from build123d import *

# Parameters (mm, degrees)
BOSS_EXTRUDE1_DEPTH                            = 27.5
CBORE_FOR_M3_SBHCS1_D                          = 3.4
CBORE_FOR_M3_SBHCS1_DEPTH                      = 14.9999954
CBORE_FOR_M3_SBHCS1_CBORE_D                    = 6.7
CBORE_FOR_M3_SBHCS1_CBORE_DEPTH                = 1.65
CBORE_FOR_M3_SBHCS1_TIP                        = 1.021463052
SKETCH4_W                                      = 41.25
SKETCH4_H                                      = 7.273611758
BOSS_EXTRUDE2_DEPTH                            = 4.5
CSK_FOR_M5_FLAT_HEAD_MACHINE_SCREW1_AT_2_COUNT = 2
CSK_FOR_M5_FLAT_HEAD_MACHINE_SCREW1_AT_2_PITCH = 32
CSK_FOR_M5_FLAT_HEAD_MACHINE_SCREW1_AT_3_COUNT = 2
CSK_FOR_M5_FLAT_HEAD_MACHINE_SCREW1_AT_3_PITCH = 43.863424399
CSK_FOR_M5_FLAT_HEAD_MACHINE_SCREW1_AT_4_COUNT = 2
CSK_FOR_M5_FLAT_HEAD_MACHINE_SCREW1_AT_4_PITCH = 30
CUT_EXTRUDE1_REACH                             = 136.892
CUT_EXTRUDE1_END_RADIUS                        = 57.15
SKETCH13_R                                     = 5.2
CHAMFER1_START                                 = -27.5
CHAMFER1_DEPTH                                 = 55
CHAMFER1_START_2                               = -3.038209282
CHAMFER1_2_OUTLINE_R                           = 3.35
CHAMFER1_2_DEPTH                               = 1.570474688
CHAMFER2_SIZE                                  = 1


with BuildPart() as part:
    # Sketch1 → Boss-Extrude1 (new, symmetric)
    with BuildSketch(Plane(origin=(0, 0, 0), x_dir=(1, 0, 0), z_dir=(0, 1, 0))):
        with BuildLine():
            Line((-25.625, 54.611949242), (-25.625, 69.598611758))
            Line((-25.625, 69.598611758), (-20.625, 69.598611758))
            Line((-20.625, 69.598611758), (-20.625, 62.325))
            Line((-20.625, 62.325), (20.625, 62.325))
            Line((20.625, 62.325), (20.625, 69.598611758))
            Line((20.625, 69.598611758), (25.625, 69.598611758))
            Line((25.625, 69.598611758), (28.64505971, 67.064480768))
            Line((28.64505971, 67.064480768), (21.893060118, 59.017760997))
            Line((21.893060118, 59.017760997), (25.723282334, 55.803822949))
            Line((25.723282334, 55.803822949), (32.475281926, 63.85054272))
            Line((32.475281926, 63.85054272), (36.305504142, 60.636604672))
            Line((36.305504142, 60.636604672), (29.553504549, 52.5898849))
            Line((29.553504549, 52.5898849), (31.287947409, 47.824542307))
            ThreePointArc((31.287947409, 47.824542307), (-32.73018113, -46.849308887), (34.142039673, 45.830597061))
            Line((34.142039673, 45.830597061), (32.272757303, 50.966408163))
            Line((32.272757303, 50.966408163), (38.7006334, 58.626852595))
            Line((38.7006334, 58.626852595), (42.530855615, 55.412914546))
            Line((42.530855615, 55.412914546), (36.399549462, 48.10590841))
            ThreePointArc((36.399549462, 48.10590841), (-6.293240092, -59.995839474), (-25.625, 54.611949242))
        make_face()
    extrude(amount=BOSS_EXTRUDE1_DEPTH, both=True)

    # CBORE for M3 SBHCS1
    with Locations(Plane(origin=(-2.327403337, 0, -1.952923282), x_dir=(0.6427876096865344, 0, -0.7660444431189822), z_dir=(0.7660444431189822, 0, 0.6427876096865344))):
        with Locations((65.056031142, 20), (65.056031142, 0), (65.056031142, -20)):
            CounterBoreHole(CBORE_FOR_M3_SBHCS1_D / 2, CBORE_FOR_M3_SBHCS1_CBORE_D / 2, CBORE_FOR_M3_SBHCS1_CBORE_DEPTH, depth=CBORE_FOR_M3_SBHCS1_DEPTH)
            with Locations((0, 0, -(CBORE_FOR_M3_SBHCS1_DEPTH + CBORE_FOR_M3_SBHCS1_TIP / 2))):  # 118° drill point
                Cone(0, CBORE_FOR_M3_SBHCS1_D / 2, CBORE_FOR_M3_SBHCS1_TIP, mode=Mode.SUBTRACT)

    # Sketch4 → Boss-Extrude2 (add)
    with BuildSketch(Plane.XZ.offset(-27.5)):
        with Locations((0, -65.961805879)):
            Rectangle(SKETCH4_W, SKETCH4_H)
    extrude(amount=BOSS_EXTRUDE2_DEPTH)

    # Sketch12 → CSK for M5 Flat Head Machine Screw1 (revolve, cut)
    with BuildSketch(Plane(origin=(-16, 15, -57.15), x_dir=(0, -1, 0), z_dir=(1, 0, 0))):
        Polygon((0, 0), (0, 12.448611758), (2.75, 12.448611758), (2.75, 2.45), (5.2, 0), align=None)
    csk_for_m5_flat_head_machine_screw1 = revolve(axis=Axis((-16, 15, -50.8), (0, 0, -1)), mode=Mode.SUBTRACT)

    # CSK for M5 Flat Head Machine Screw1 at 2: CSK for M5 Flat Head Machine Screw1 ×2
    with Locations(*[(i * CSK_FOR_M5_FLAT_HEAD_MACHINE_SCREW1_AT_2_PITCH, 0, 0) for i in range(1, CSK_FOR_M5_FLAT_HEAD_MACHINE_SCREW1_AT_2_COUNT)]):
        add(csk_for_m5_flat_head_machine_screw1, mode=Mode.SUBTRACT)

    # CSK for M5 Flat Head Machine Screw1 at 3: CSK for M5 Flat Head Machine Screw1 ×2
    with Locations(*[Vector(0.7295372041400852, -0.6839411288813297, 0) * (i * CSK_FOR_M5_FLAT_HEAD_MACHINE_SCREW1_AT_3_PITCH) for i in range(1, CSK_FOR_M5_FLAT_HEAD_MACHINE_SCREW1_AT_3_COUNT)]):
        add(csk_for_m5_flat_head_machine_screw1, mode=Mode.SUBTRACT)

    # CSK for M5 Flat Head Machine Screw1 at 4: CSK for M5 Flat Head Machine Screw1 ×2
    with Locations(*[(0, -i * CSK_FOR_M5_FLAT_HEAD_MACHINE_SCREW1_AT_4_PITCH, 0) for i in range(1, CSK_FOR_M5_FLAT_HEAD_MACHINE_SCREW1_AT_4_COUNT)]):
        add(csk_for_m5_flat_head_machine_screw1, mode=Mode.SUBTRACT)

    # Cut-Extrude1: up to this cylinder (the profile starts outside it)
    cut_extrude1_end = Plane(origin=(0, 0, 0), z_dir=(0, -1, 0)) * Cylinder(CUT_EXTRUDE1_END_RADIUS, 419.084, mode=Mode.PRIVATE)
    # Sketch13 → Cut-Extrude1 (cut, up to the surface)
    with BuildSketch(Plane.XY.offset(-57.15), mode=Mode.PRIVATE) as cut_extrude1_sk1:
        with Locations(Location((-16, -15, 0), (0, 0, 180))):
            Circle(SKETCH13_R)
    cut_extrude1_tool1 = extrude(cut_extrude1_sk1.sketch, amount=CUT_EXTRUDE1_REACH, mode=Mode.PRIVATE) - cut_extrude1_end
    add(cut_extrude1_tool1.solids().sort_by_distance((-16, -15, -57.15))[0], mode=Mode.SUBTRACT)
    # Sketch13 → Cut-Extrude1 (cut, up to the surface)
    with BuildSketch(Plane.XY.offset(-57.15), mode=Mode.PRIVATE) as cut_extrude1_sk2:
        with Locations(Location((16, -15, 0), (0, 0, 180))):
            Circle(SKETCH13_R)
    cut_extrude1_tool2 = extrude(cut_extrude1_sk2.sketch, amount=CUT_EXTRUDE1_REACH, mode=Mode.PRIVATE) - cut_extrude1_end
    add(cut_extrude1_tool2.solids().sort_by_distance((16, -15, -57.15))[0], mode=Mode.SUBTRACT)
    # Sketch13 → Cut-Extrude1 (cut, up to the surface)
    with BuildSketch(Plane.XY.offset(-57.15), mode=Mode.PRIVATE) as cut_extrude1_sk3:
        with Locations(Location((16, 15, 0), (0, 0, 180))):
            Circle(SKETCH13_R)
    cut_extrude1_tool3 = extrude(cut_extrude1_sk3.sketch, amount=CUT_EXTRUDE1_REACH, mode=Mode.PRIVATE) - cut_extrude1_end
    add(cut_extrude1_tool3.solids().sort_by_distance((16, 15, -57.15))[0], mode=Mode.SUBTRACT)
    # Sketch13 → Cut-Extrude1 (cut, up to the surface)
    with BuildSketch(Plane.XY.offset(-57.15), mode=Mode.PRIVATE) as cut_extrude1_sk4:
        with Locations(Location((-16, 15, 0), (0, 0, 180))):
            Circle(SKETCH13_R)
    cut_extrude1_tool4 = extrude(cut_extrude1_sk4.sketch, amount=CUT_EXTRUDE1_REACH, mode=Mode.PRIVATE) - cut_extrude1_end
    add(cut_extrude1_tool4.solids().sort_by_distance((-16, 15, -57.15))[0], mode=Mode.SUBTRACT)

    # Chamfer1: read off the stored shape, not the designer's step
    # Chamfer1 outline → Chamfer1 (add)
    with BuildSketch(Plane(origin=(0, 0, 0), x_dir=(1, 0, 0), z_dir=(0, 1, 0)).offset(CHAMFER1_START)):
        with BuildLine():
            ThreePointArc((36.399549462, 48.10590841), (37.595386052, 47.177246344), (38.767539596, 46.218865181))
            Line((38.767539596, 46.218865181), (38.293658487, 50.363219646))
            Line((38.293658487, 50.363219646), (36.399549462, 48.10590841))
        make_face()
        with BuildLine():
            Line((-25.625, 57.786949242), (-32.752511971, 50.659437271))
            ThreePointArc((-32.752511971, 50.659437271), (-29.255581753, 52.756199269), (-25.625, 54.611949242))
            Line((-25.625, 54.611949242), (-25.625, 57.786949242))
        make_face()
    extrude(amount=CHAMFER1_DEPTH)

    # Chamfer1 2 outline → Chamfer1 2 (cut)
    with BuildSketch(Plane(origin=(0, 0, 0), x_dir=(0.642787609686534, 0, -0.7660444431189825), z_dir=(0.7660444431189823, 0, 0.6427876096865344)).offset(CHAMFER1_START_2)):
        with Locations((65.056031142, -20)):
            Circle(CHAMFER1_2_OUTLINE_R)
        with Locations((65.056031142, 0)):
            Circle(CHAMFER1_2_OUTLINE_R)
        with Locations((65.056031142, 20)):
            Circle(CHAMFER1_2_OUTLINE_R)
    extrude(amount=CHAMFER1_2_DEPTH, mode=Mode.SUBTRACT)

    # Chamfer2
    chamfer2_edges = [part.edges().sort_by_distance(p)[0] for p in [
        (21.893060118, 0, -59.017760997),
        (25.723282334, 0, -55.803822949),
    ]]
    chamfer(chamfer2_edges, length=CHAMFER2_SIZE)


solid = part.part
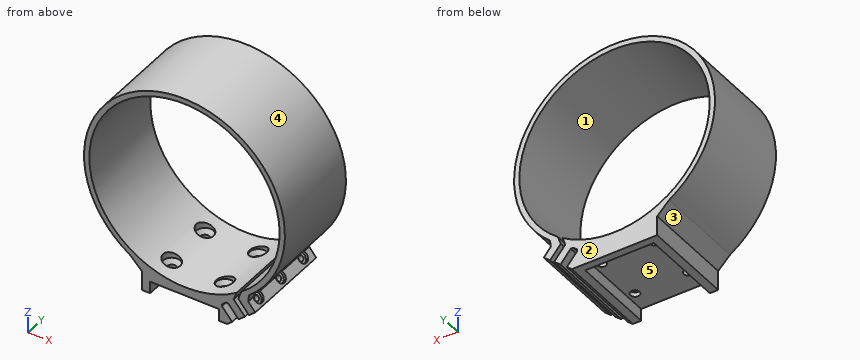
Check sheet for the modelled part. Datum: model origin and axes. Units: mm. Face numbers are marked on the shaded views. A direction names the side the tool comes from. Round coordinates to 2 decimals unless told otherwise and drop trailing zeros. Loops run counter-clockwise (first coordinate to the right, second up) from the corner with the lowest first, then second, coordinate; pieces in that order, holes last.
1. Set-up check for the marked faces 4 and 5: record each of +Z, -Z, +X, -X, +Y, -Y from which the full face is reachable in a straight line by a thin tool's end or side.
2. Mould release check, pull along X, two halves, no side actions. Record for the marked faces 1, 2 and 3: released by +X, released by -X, zero draft, split by the parting line, or undercut.
3. Sectioned sample at D-D on x = -16. Record the boundary of the cut face in (y, z) (3 decimals), and give its area (3 significant figures).
4. Sectioned sample at B-B on z = -11.5. Record the boundary of the cut face in (x, y).
5. Gauge pin test, flat ends, axial feed: pin 1 Ø4 at (y, z) = (11.5, 29) entering from +X; pin 2 Ø6 at (x, y) = (-16, 15) entering from +Z; pin 3 Ø12.5 at (x, y) = (-7, 3.5) entering from -Z (3 decimals); pin 4 Ø3 at (x, y) = (19.5, 4) entering from -Z. Record the tip position at first contact, or that the pin passes through.
6. Sectioned sample at C-C on x = -51.5. Record the boundary of the cut face in (y, z), and give its area (3 significant figures).
7. Scan lines: probe 1 along Y at (x, z) = (16, -55.5); probe 2 along Y at (x, z) = (-16, -60.45); probe 3 along X at (y, z) = (15, -54.1). Record each from-to range of solid material in increasing order.
Recorded:
1. face 4: +Y, -Y
1. face 5: -Z, -Y
2. face 1: undercut
2. face 2: zero draft
2. face 3: released by -X
3. outline: (-27.5, -62.325) - (-17.75, -62.325) - (-17.75, -59.6) - (-20.2, -57.15) - (-20.2, -54.865) - (-27.5, -54.865) - close; (-27.5, 54.865) - (27.5, 54.865) - (27.5, 58.164) - (-27.5, 58.164) - close; (-12.25, -62.325) - (12.25, -62.325) - (12.25, -59.6) - (9.8, -57.15) - (9.8, -54.865) - (-9.8, -54.865) - (-9.8, -57.15) - (-12.25, -59.6) - close; (17.75, -62.325) - (23, -62.325) - (23, -69.599) - (27.5, -69.599) - (27.5, -54.865) - (20.2, -54.865) - (20.2, -57.15) - (17.75, -59.6) - close
3. area: 508 mm2
4. outline: (-59.22, -27.5) - (-55.98, -27.5) - (-55.98, 27.5) - (-59.22, 27.5) - close; (55.98, -27.5) - (59.22, -27.5) - (59.22, 27.5) - (55.98, 27.5) - close
5. pin 1: stops at x = 53.95
5. pin 2: stops at z = 58.91
5. pin 3: stops at z = -62.325
5. pin 4: stops at z = -69.6
6. outline: (-27.5, -31.41) - (27.5, -31.41) - (27.5, -24.78) - (-27.5, -24.78) - close; (-27.5, 24.78) - (27.5, 24.78) - (27.5, 31.41) - (-27.5, 31.41) - close
6. area: 730 mm2
7. probe 1: y = -27.5 to -20.2, -9.8 to 9.8, 20.2 to 27.5
7. probe 2: y = -27.5 to -17.75, -12.25 to 12.25, 17.75 to 27.5
7. probe 3: x = -29.31 to -21.2, 21.2 to 30.82, 34.9 to 41.43
